Can you work these out from the model? Positions are in its coordinate system, mm. Face numbers are marked on the shaded views. Give positions to 0.01 mm unless a question says otherwise; leave off trailing zeros. Loops run counter-clockwise (first coordinate to the right, second up) from the corner with the lowest first, then second, coordinate; pieces in that order, holes last. Notation, with made-up numbers: M 81,36 L 116,36 A23 ccw 116,70 Z; hole C -1.75,54 d2. An arc over 180 degrees is marked long. One line per item, written item: value. Start each with the question number.
from build123d import *

# Parameters (mm, degrees)
SKETCH1_W                = 175
SKETCH1_H                = 200
BOSS_EXTRUDE1_DEPTH      = 10
SKETCH3_W                = 5
SKETCH3_H                = 25
SKETCH3_W_2              = 25
SKETCH3_H_2              = 5
BOSS_EXTRUDE2_DEPTH      = 25
CHAMFER1_SIZE            = 25
SKETCH4_R                = 3.5
SKETCH4_R_2              = 1.25
CUT_EXTRUDE1_DEPTH       = 25
CHAMFER1_OF_MIRROR1_SIZE = 25
SKETCH5_R                = 5
CUT_EXTRUDE2_DEPTH       = 10
SKETCH6_R                = 1.5
CUT_EXTRUDE3_DEPTH       = 10


# Read off the part's stored shape, not the designer's step: Mirror2
with BuildPart() as part:
    # Sketch1 → Boss-Extrude1 (new body)
    with BuildSketch(Plane(origin=(0, 0, 0), x_dir=(1, 0, 0), z_dir=(0, 1, 0))):
        with Locations((87.5, 100)):
            Rectangle(SKETCH1_W, SKETCH1_H)
    extrude(amount=BOSS_EXTRUDE1_DEPTH)

    # Sketch3 → Boss-Extrude2 (add)
    with BuildSketch(Plane(origin=(0, 10, 0), x_dir=(1, 0, 0), z_dir=(0, 1, 0))):
        with Locations((2.5, 72.5)):
            Rectangle(SKETCH3_W, SKETCH3_H)
        Polygon((0, 60), (0, 25), (5, 25), (5, 30), (5, 55), (5, 60), align=None)
        with Locations((17.5, 57.5)):
            Rectangle(SKETCH3_W_2, SKETCH3_H_2)
        with Locations((17.5, 27.5)):
            Rectangle(SKETCH3_W_2, SKETCH3_H_2)
        with Locations((2.5, 12.5)):
            Rectangle(SKETCH3_W, SKETCH3_H)
    boss_extrude2 = extrude(amount=BOSS_EXTRUDE2_DEPTH)

    # Chamfer1
    chamfer1_edges = [part.edges().sort_by_distance(p)[0] for p in [
        (2.5, 35, -85),
        (30, 35, -57.5),
        (30, 35, -27.5),
        (2.5, 35, 0),
    ]]
    chamfer(chamfer1_edges, length=CHAMFER1_SIZE - 0.0001)  # a hair under: the kernel refuses the full size

    # Sketch4 → Cut-Extrude1 (cut)
    with BuildSketch(Plane(origin=(5, 0, 0), x_dir=(0, 0, -1), z_dir=(1, 0, 0))):
        with Locations((42.5, 22.5)):
            Circle(SKETCH4_R)
        with Locations((34, 22.5)):
            Circle(SKETCH4_R_2)
        with Locations((51, 22.5)):
            Circle(SKETCH4_R_2)
    cut_extrude1 = extrude(amount=-CUT_EXTRUDE1_DEPTH, mode=Mode.SUBTRACT)

    # Mirror1: Boss-Extrude2, Cut-Extrude1 across plane
    add(boss_extrude2.mirror(Plane(origin=(87.5, 0, 0), x_dir=(0, 0, 1), z_dir=(1, 0, 0))))
    add(cut_extrude1.mirror(Plane(origin=(87.5, 0, 0), x_dir=(0, 0, 1), z_dir=(1, 0, 0))), mode=Mode.SUBTRACT)

    # Chamfer1 of Mirror1
    chamfer1_of_mirror1_edges = [part.edges().sort_by_distance(p)[0] for p in [
        (172.5, 35, -85),
        (145, 35, -57.5),
        (145, 35, -27.5),
        (172.5, 35, 0),
    ]]
    chamfer(chamfer1_of_mirror1_edges, length=CHAMFER1_OF_MIRROR1_SIZE - 0.0001)  # a hair under: the kernel refuses the full size

    # Mirror2: part across plane


with BuildPart() as part_1:
    add(part.part)
    add(part.part.mirror(Plane.XY.offset(-100)))

    # Sketch5 → Cut-Extrude2 (cut)
    with BuildSketch(Plane(origin=(0, 10, 0), x_dir=(1, 0, 0), z_dir=(0, 1, 0))):
        with Locations(Location((87.5, 100, 0), (0, 0, 270))):
            Circle(SKETCH5_R)
    extrude(amount=-CUT_EXTRUDE2_DEPTH, mode=Mode.SUBTRACT)

    # Sketch6 → Cut-Extrude3 (cut)
    with BuildSketch(Plane.XZ):
        with Locations(Location((15, -71, 0), (0, 0, 270))):
            Circle(SKETCH6_R)
        with Locations(Location((64, -71, 0), (0, 0, 270))):
            Circle(SKETCH6_R)
        with Locations(Location((15, -129, 0), (0, 0, 270))):
            Circle(SKETCH6_R)
        with Locations(Location((64, -129, 0), (0, 0, 270))):
            Circle(SKETCH6_R)
    extrude(amount=-CUT_EXTRUDE3_DEPTH, mode=Mode.SUBTRACT)


solid = part_1.part
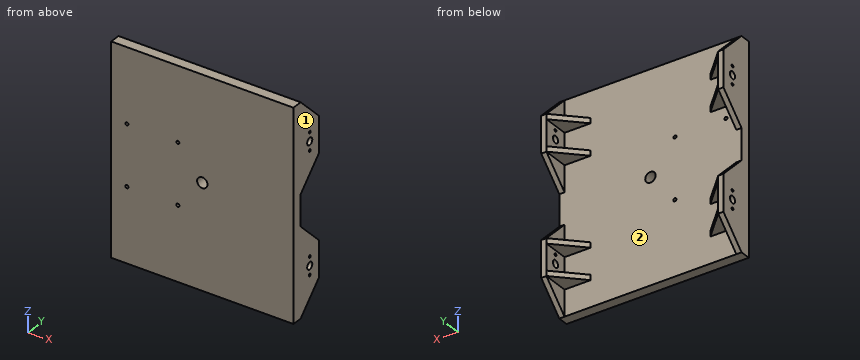
Q1. If we section it at D-D, the plane x = 150: Write out the boundary of the cut face in (y, z), plus the area to 3 significant figures.
Q2. If we mould it in two halves opening along Z, with no side actions, what happens to the marked faces 1 and 2? For each: released by +Z, released by -Z, zero draft, split by the parting line, or undercut.
Q3. I need wall thicknesses on line 1 along Z through (x, y) = (161, 14); line 2 along X through (y, z) = (14.5, -74); line 3 along Y through (x, z) = (173.5, -51). Which ranges of each line are inside material? Lowest first, please.
Q4. If we section it at C-C, the plane y = 16: Give the number of separate pieces and of enclosed holes in the cut face, plus the area to 3 significant figures.
Q5. If we section it at A-A, the plane z = -42.5: Write out the boundary of the cut face in (x, y).
Q6. For P1, Ø4, axis at x = 64, z = -129, coming from the -Y side; P2, Ø20, axis at x = 157.5, y = 22, coming from the -Z side; P3, Ø12.5, axis at x = 18, y = 22, coming from the +Z side; P4, Ø20, axis at x = 13, y = 25.5, coming from the +Z side, each with a flat end and sliding along its axis, tell me the tip position at first contact or that it passes through.
Q7. If we section it at B-B, the plane x = 47: Write out the boundary of the cut face in (y, z).
Response:
1. outline: M 0,-200 L 10,-200 L 10,-175 L 15,-175 L 15,-170 L 10,-170 L 10,-145 L 15,-145 L 15,-140 L 10,-140 L 10,-60 L 15,-60 L 15,-55 L 10,-55 L 10,-30 L 15,-30 L 15,-25 L 10,-25 L 10,0 L 0,0 Z
1. area: 2,100 mm^2
2. face 1: zero draft
2. face 2: undercut
3. line 1: -175 to -170, -145 to -140, -60 to -55, -30 to -25
3. line 2: 0 to 5, 170 to 175
3. line 3: 0 to 21.25, 23.75 to 35
4. separate pieces: 4
4. enclosed holes: 0
4. area: 2,220 mm^2
5. outline: M 0,0 L 175,0 L 175,19 L 170,19 L 170,10 L 5,10 L 5,19 L 0,19 Z; M 0,26 L 5,26 L 5,35 L 0,35 Z; M 170,26 L 175,26 L 175,35 L 170,35 Z
6. P1: y = 0
6. P2: z = -175
6. P3: z = -25
6. P4: z = -9.5
7. outline: M 0,-200 L 10,-200 L 10,0 L 0,0 Z
